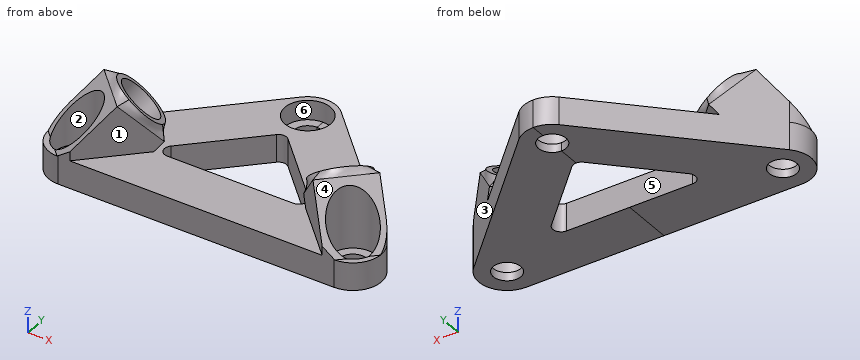
from build123d import *
from build123d.topology import SkipClean

# Parameters (mm, degrees)
BOSS_EXTRUDE1_DEPTH = 10
SKETCH2_R           = 8.25
CUT_EXTRUDE1_DEPTH  = 7
CUT_EXTRUDE2_DEPTH  = 16
FILLET2_R           = 3
SKETCH5_R           = 5
CUT_EXTRUDE3_DEPTH  = 16
BOSS_EXTRUDE2_DEPTH = 20.5
CUT_EXTRUDE4_START  = 20
SKETCH7_R           = 8.25
SKETCH7_R_2         = 5
CUT_EXTRUDE4_DEPTH  = 20
SKETCH9_R           = 8.25
CUT_EXTRUDE5_DEPTH  = 5
SKETCH10_W          = 60.25
SKETCH10_H          = 70.5
CUT_EXTRUDE6_DEPTH  = 45


with BuildPart() as part:
    # Sketch1 → Boss-Extrude1 (new body)
    with BuildSketch(Plane.XY):
        with BuildLine():
            Line((0, 10.25), (100, 10.25))
            ThreePointArc((100, 10.25), (110.25, 0), (100, -10.25))
            Line((100, -10.25), (0, -10.25))
            ThreePointArc((0, -10.25), (-10.25, 0), (0, 10.25))
        make_face()
        with BuildLine():
            Line((92.752155493, -7.247844507), (42.752155493, 42.752155493))
            ThreePointArc((42.752155493, 42.752155493), (42.752155493, 57.247844507), (57.247844507, 57.247844507))
            Line((57.247844507, 57.247844507), (107.247844507, 7.247844507))
            ThreePointArc((107.247844507, 7.247844507), (107.247844507, -7.247844507), (92.752155493, -7.247844507))
        make_face()
        with BuildLine():
            Line((57.247844507, 42.752155493), (7.247844507, -7.247844507))
            ThreePointArc((7.247844507, -7.247844507), (-7.247844507, -7.247844507), (-7.247844507, 7.247844507))
            Line((-7.247844507, 7.247844507), (42.752155493, 57.247844507))
            ThreePointArc((42.752155493, 57.247844507), (57.247844507, 57.247844507), (57.247844507, 42.752155493))
        make_face()
    extrude(amount=BOSS_EXTRUDE1_DEPTH)

    # Sketch2 → Cut-Extrude1 (cut)
    with BuildSketch(Plane.XY.offset(10)):
        with Locations((50, 50)):
            Circle(SKETCH2_R)
        with Locations((100, 0)):
            Circle(SKETCH2_R)
        Circle(SKETCH2_R)
    extrude(amount=-CUT_EXTRUDE1_DEPTH, mode=Mode.SUBTRACT)

    # Sketch4 → Cut-Extrude2 (cut)
    with BuildSketch(Plane.XY.offset(10)):
        Polygon((19.91726189, 8.25), (80.08273811, 8.25), (50, 38.33273811), align=None)
    extrude(amount=-CUT_EXTRUDE2_DEPTH, mode=Mode.SUBTRACT)

    # Fillet2
    fillet2_edges = [part.edges().sort_by_distance(p)[0] for p in [
        (19.91726189, 8.25, 5),
        (50, 38.33273811, 5),
        (80.08273811, 8.25, 5),
    ]]
    fillet(fillet2_edges, radius=FILLET2_R)

    # Sketch5 → Cut-Extrude3 (cut)
    with BuildSketch(Plane.XY.offset(10)):
        Circle(SKETCH5_R)
        with Locations((50, 50)):
            Circle(SKETCH5_R)
        with Locations((100, 0)):
            Circle(SKETCH5_R)
    extrude(amount=-CUT_EXTRUDE3_DEPTH, mode=Mode.SUBTRACT)

    # Sketch6 → Boss-Extrude2 (add)
    with BuildSketch(Plane(origin=(-7.247844507, 7.247844507, 0), x_dir=(0, 0, 1), z_dir=(-0.7071067811865441, 0.7071067811865509, 0))):
        Polygon((10, 21.495689014), (10, 7), (20.500892834, 17.500892834), (13.253048327, 24.748737342), align=None)
        Polygon((20.500892834, 17.500892834), (10, 7), (10, 0), (10, -7.495689014), (27.748737342, 10.253048327), align=None)
    extrude(amount=-BOSS_EXTRUDE2_DEPTH)

    # Sketch7 → Cut-Extrude4 (cut)
    # profile 1 of 3: a face of its own
    with BuildSketch(Plane.XY.offset(10).offset(CUT_EXTRUDE4_START)):
        with BuildLine():
            Line((20, -20.25), (20, -10.25))
            Line((20, -10.25), (4.245689014, -10.25))
            Line((4.245689014, -10.25), (0, -10.25))
            ThreePointArc((0, -10.25), (-9.469765208, -3.922505182), (-7.247844507, 7.247844507))
            Line((-7.247844507, 7.247844507), (7.951902961, 22.447591975))
            Line((7.951902961, 22.447591975), (15.254310986, 29.75))
            Line((15.254310986, 29.75), (-20, 29.75))
            Line((-20, 29.75), (-20, -20.25))
            Line((-20, -20.25), (20, -20.25))
        make_face()
    # profile 2 of 3: a face of its own
    with BuildSketch(Plane.XY.offset(10).offset(CUT_EXTRUDE4_START)):
        Circle(SKETCH7_R)
        Circle(SKETCH7_R_2, mode=Mode.SUBTRACT)
    # profile 3 of 3: a face of its own
    with BuildSketch(Plane.XY.offset(10).offset(CUT_EXTRUDE4_START)):
        Circle(SKETCH7_R_2)
    extrude(amount=-CUT_EXTRUDE4_DEPTH, mode=Mode.SUBTRACT)

    # Loft1: read off the stored shape, not the designer's step
    # Loft1: loft between two sections, ruled curve by curve
    loft1_from = [
        Edge.make_bspline([(12.373922254, 22.623922254, 17.497213178), (12.889457441, 22.535470399, 17.195219657), (13.432134989, 22.397880865, 16.908779176), (14.549790596, 22.011562197, 16.391645867), (15.124688663, 21.762676267, 16.161120474), (16.274806274, 21.151537295, 15.780005023), (16.849824782, 20.789221108, 15.629601769), (17.962375724, 19.963587433, 15.426720624), (18.499640751, 19.500359249, 15.374368671), (19.500359249, 18.499640751, 15.374368671), (19.963587433, 17.962375724, 15.426720624), (20.789221108, 16.849824782, 15.629601769), (21.151537295, 16.274806274, 15.780005023), (21.762676267, 15.124688663, 16.161120474), (22.011562197, 14.549790596, 16.391645867), (22.397880865, 13.432134989, 16.908779176), (22.535470399, 12.889457441, 17.195219657), (22.623922254, 12.373922254, 17.497213178)], [0, 0, 0, 0, 0.125, 0.125, 0.25, 0.25, 0.375, 0.375, 0.5, 0.5, 0.625, 0.625, 0.75, 0.75, 0.875, 0.875, 1, 1, 1, 1], 3),
        Edge.make_bspline([(22.623922254, 12.373922254, 17.497213178), (22.712374108, 11.858387066, 17.799206699), (22.758303856, 11.331435851, 18.13934024), (22.743701961, 10.282567338, 18.891327377), (22.682975729, 9.76079032, 19.303219376), (22.441392942, 8.756976633, 20.183847667), (22.260398337, 8.27517552, 20.652515015), (21.778027739, 7.387042631, 21.621607323), (21.476651925, 6.980962911, 22.121853929), (20.769037089, 6.273348075, 23.122572427), (20.362957369, 5.971972261, 23.622819032), (19.47482448, 5.489601663, 24.591911341), (18.993023367, 5.308607058, 25.060578689), (17.98920968, 5.067024271, 25.94120698), (17.467432662, 5.006298039, 26.353098979), (16.418564149, 4.991696144, 27.105086116), (15.891612934, 5.037625892, 27.445219657), (15.376077746, 5.126077746, 27.747213178)], [0, 0, 0, 0, 0.125, 0.125, 0.25, 0.25, 0.375, 0.375, 0.5, 0.5, 0.625, 0.625, 0.75, 0.75, 0.875, 0.875, 1, 1, 1, 1], 3),
        Edge.make_bspline([(5.126077746, 15.376077746, 27.747213178), (5.037625892, 15.891612934, 27.445219657), (4.991696144, 16.418564149, 27.105086116), (5.006298039, 17.467432662, 26.353098979), (5.067024271, 17.98920968, 25.94120698), (5.308607058, 18.993023367, 25.060578689), (5.489601663, 19.47482448, 24.591911341), (5.971972261, 20.362957369, 23.622819032), (6.273348075, 20.769037089, 23.122572427), (6.980962911, 21.476651925, 22.121853929), (7.387042631, 21.778027739, 21.621607323), (8.27517552, 22.260398337, 20.652515015), (8.756976633, 22.441392942, 20.183847667), (9.76079032, 22.682975729, 19.303219376), (10.282567338, 22.743701961, 18.891327377), (11.331435851, 22.758303856, 18.13934024), (11.858387066, 22.712374108, 17.799206699), (12.373922254, 22.623922254, 17.497213178)], [0, 0, 0, 0, 0.125, 0.125, 0.25, 0.25, 0.375, 0.375, 0.5, 0.5, 0.625, 0.625, 0.75, 0.75, 0.875, 0.875, 1, 1, 1, 1], 3),
        Edge.make_bspline([(15.376077746, 5.126077746, 27.747213178), (14.860542559, 5.214529601, 28.049206699), (14.317865011, 5.352119135, 28.33564718), (13.200209404, 5.738437803, 28.852780489), (12.625311337, 5.987323733, 29.083305882), (11.475193726, 6.598462705, 29.464421332), (10.900175218, 6.960778892, 29.614824586), (9.787624276, 7.786412567, 29.817705732), (9.250359249, 8.249640751, 29.870057685), (8.249640751, 9.250359249, 29.870057685), (7.786412567, 9.787624276, 29.817705732), (6.960778892, 10.900175218, 29.614824586), (6.598462705, 11.475193726, 29.464421332), (5.987323733, 12.625311337, 29.083305882), (5.738437803, 13.200209404, 28.852780489), (5.352119135, 14.317865011, 28.33564718), (5.214529601, 14.860542559, 28.049206699), (5.126077746, 15.376077746, 27.747213178)], [0, 0, 0, 0, 0.125, 0.125, 0.25, 0.25, 0.375, 0.375, 0.5, 0.5, 0.625, 0.625, 0.75, 0.75, 0.875, 0.875, 1, 1, 1, 1], 3),
    ]
    loft1_to = [
        Edge.make_bspline([(10.252155493, 24.747844507, 13.253048327), (10.856142535, 24.143857465, 13.253048327), (11.460129577, 23.539870423, 13.253048327), (12.668103662, 22.331896338, 13.253048327), (13.272090704, 21.727909296, 13.253048327), (14.480064789, 20.519935211, 13.253048327), (15.084051831, 19.915948169, 13.253048327), (16.292025915, 18.707974085, 13.253048327), (16.896012958, 18.103987042, 13.253048327), (18.103987042, 16.896012958, 13.253048327), (18.707974085, 16.292025915, 13.253048327), (19.915948169, 15.084051831, 13.253048327), (20.519935211, 14.480064789, 13.253048327), (21.727909296, 13.272090704, 13.253048327), (22.331896338, 12.668103662, 13.253048327), (23.539870423, 11.460129577, 13.253048327), (24.143857465, 10.856142535, 13.253048327), (24.747844507, 10.252155493, 13.253048327)], [0, 0, 0, 0, 0.125, 0.125, 0.25, 0.25, 0.375, 0.375, 0.5, 0.5, 0.625, 0.625, 0.75, 0.75, 0.875, 0.875, 1, 1, 1, 1], 3),
        Edge.make_bspline([(24.747844507, 10.252155493, 13.253048327), (24.320761174, 9.82507216, 13.857035369), (23.89367784, 9.397988826, 14.461022412), (23.039511174, 8.54382216, 15.668996496), (22.61242784, 8.116738826, 16.272983539), (21.758261174, 7.26257216, 17.480957623), (21.33117784, 6.835488826, 18.084944665), (20.477011174, 5.98132216, 19.29291875), (20.04992784, 5.554238826, 19.896905792), (19.195761174, 4.70007216, 21.104879877), (18.76867784, 4.272988826, 21.708866919), (17.914511174, 3.41882216, 22.916841003), (17.48742784, 2.991738826, 23.520828046), (16.633261174, 2.13757216, 24.72880213), (16.20617784, 1.710488826, 25.332789172), (15.352011174, 0.85632216, 26.540763257), (14.92492784, 0.429238826, 27.144750299), (14.497844507, 0.002155493, 27.748737342)], [0, 0, 0, 0, 0.125, 0.125, 0.25, 0.25, 0.375, 0.375, 0.5, 0.5, 0.625, 0.625, 0.75, 0.75, 0.875, 0.875, 1, 1, 1, 1], 3),
        Edge.make_bspline([(0.002155493, 14.497844507, 27.748737342), (0.429238826, 14.92492784, 27.144750299), (0.85632216, 15.352011174, 26.540763257), (1.710488826, 16.20617784, 25.332789172), (2.13757216, 16.633261174, 24.72880213), (2.991738826, 17.48742784, 23.520828046), (3.41882216, 17.914511174, 22.916841003), (4.272988826, 18.76867784, 21.708866919), (4.70007216, 19.195761174, 21.104879877), (5.554238826, 20.04992784, 19.896905792), (5.98132216, 20.477011174, 19.29291875), (6.835488826, 21.33117784, 18.084944665), (7.26257216, 21.758261174, 17.480957623), (8.116738826, 22.61242784, 16.272983539), (8.54382216, 23.039511174, 15.668996496), (9.397988826, 23.89367784, 14.461022412), (9.82507216, 24.320761174, 13.857035369), (10.252155493, 24.747844507, 13.253048327)], [0, 0, 0, 0, 0.125, 0.125, 0.25, 0.25, 0.375, 0.375, 0.5, 0.5, 0.625, 0.625, 0.75, 0.75, 0.875, 0.875, 1, 1, 1, 1], 3),
        Edge.make_bspline([(14.497844507, 0.002155493, 27.748737342), (13.893857465, 0.606142535, 27.748737342), (13.289870423, 1.210129577, 27.748737342), (12.081896338, 2.418103662, 27.748737342), (11.477909296, 3.022090704, 27.748737342), (10.269935211, 4.230064789, 27.748737342), (9.665948169, 4.834051831, 27.748737342), (8.457974085, 6.042025915, 27.748737342), (7.853987042, 6.646012958, 27.748737342), (6.646012958, 7.853987042, 27.748737342), (6.042025915, 8.457974085, 27.748737342), (4.834051831, 9.665948169, 27.748737342), (4.230064789, 10.269935211, 27.748737342), (3.022090704, 11.477909296, 27.748737342), (2.418103662, 12.081896338, 27.748737342), (1.210129577, 13.289870423, 27.748737342), (0.606142535, 13.893857465, 27.748737342), (0.002155493, 14.497844507, 27.748737342)], [0, 0, 0, 0, 0.125, 0.125, 0.25, 0.25, 0.375, 0.375, 0.5, 0.5, 0.625, 0.625, 0.75, 0.75, 0.875, 0.875, 1, 1, 1, 1], 3),
    ]
    loft1 = Solid(Shell([*[Face.make_surface_from_curves(loft1_from[k], loft1_to[k]) for k in range(4)], Face(Wire(loft1_from)), Face(Wire(loft1_to))]))
    add(loft1)

    # Sketch9 → Cut-Extrude5 (cut)
    with BuildSketch(Plane(origin=(14.935660172, 14.935660172, 21.122213178), x_dir=(0.8660254037844357, -0.2886751345948172, -0.40824829046386635), z_dir=(0.5000000000000052, 0.5000000000000007, 0.7071067811865435))):
        with Locations(Location((-1.224744871, -1.732050808, 0), (0, 0, 19.471220634))):
            Circle(SKETCH9_R)
    extrude(amount=-CUT_EXTRUDE5_DEPTH, mode=Mode.SUBTRACT)

    # Sketch10 → Cut-Extrude6 (cut)
    with BuildSketch(Plane(origin=(0, 0, 0), x_dir=(-1, 0, 0), z_dir=(0, 0, -1))):
        with Locations((-80.125, 25)):
            Rectangle(SKETCH10_W, SKETCH10_H)
    extrude(amount=-CUT_EXTRUDE6_DEPTH, mode=Mode.SUBTRACT)

    # Mirror1: part across plane


with BuildPart() as part_1:
    with SkipClean():  # the faces are left unmerged after this step: merging them gives an invalid solid
        add(part.part)
        add(part.part.mirror(Plane(origin=(50, 60.25, 45), x_dir=(0, 0, 1), z_dir=(-1, 0, 0))))


solid = part_1.part
Geometry check sheet. Reference: the model listing, model coordinates, mm. Face numbers are marked on the shaded views. A direction names the side the tool comes from. Round coordinates to 2 decimals unless told otherwise and drop trailing zeros. Loops run counter-clockwise (first coordinate to the right, second up) from the corner with the lowest first, then second, coordinate; pieces in that order, holes last.
Item 1: Cross-section at B-B on y = 34. Record the boundary of the cut face in (x, z).
Item 2: Gauge pin test, flat ends, axial feed: pin 1 (4 mm diameter, centred on x = 55.5, y = 48, fed in from +Z); pin 2 (5 mm diameter, centred on x = 106, y = -6, fed in from +Z); pin 3 (19 mm diameter, centred on x = 100, y = 0, fed in from +Z); pin 4 (6 mm diameter, centred on x = 0, y = 0, fed in from +Z). Record the tip position at first contact, or that the pin passes through.
Item 3: Cross-section at A-A on x = 67.5. Record the boundary of the cut face in (y, z), then the cut area to 3 significant figures.
Item 4: Cross-section at C-C on y = 50. Record the boundary of the cut face in (x, z).
Item 5: Access from +Z, -Z, +X, -X, +Y, -Y to the whole of each face (thin tool, end or side, straight path). Record for the marked faces 4, 5 and 6.
Item 6: Mould release check, pull along Y, two halves, no side actions. Record for the marked faces 1, 2 and 3: pulls with the +Y half, pulls with the -Y half, needs draft (parallel to the pull), parting line crosses it, or undercut.
Item 7: Thickness scan on line 1 (X direction, y = 0, z = 6); line 2 (Y direction, x = 50, z = 4.5); line 3 (Y direction, x = 100, z = 0.75). Record the ranges inside material, lowest first.
Answer sheet:
1. outline: (19.5, 0) - (45.67, 0) - (45.67, 10) - (19.5, 10) - close; (54.33, 0) - (80.5, 0) - (80.5, 10) - (54.33, 10) - close
2. pin 1: stops at z = 3
2. pin 2: stops at z = 10
2. pin 3: stops at z = 27
2. pin 4: passes through
3. outline: (-10.25, 0) - (8.25, 0) - (8.25, 10) - (-10.25, 10) - close; (20.83, 0) - (47, 0) - (47, 10) - (20.83, 10) - close
3. area: 447 mm2
4. outline: (35.5, 0) - (45, 0) - (45, 3) - (41.75, 3) - (41.75, 10) - (35.5, 10) - close; (55, 0) - (64.5, 0) - (64.5, 10) - (58.25, 10) - (58.25, 3) - (55, 3) - close
5. face 4: +Z, +X, -Y
5. face 5: +Z, -Z
5. face 6: +Z
6. face 1: pulls with the -Y half
6. face 2: undercut
6. face 3: pulls with the +Y half
7. line 1: x = -10.25 to -8.25, 8.25 to 91.75, 108.25 to 110.25
7. line 2: y = -10.25 to 8.25, 37.09 to 41.75, 58.25 to 60.25
7. line 3: y = -10.25 to -5, 5 to 14.5
